Can you work these out from the model? Positions are in its coordinate system, mm. Coordinates: 2 decimals unless noted, no trailing zeros. Order: outer loops, then holes, each group sorted by start corner. A loop starts at its lowest first (then second) coordinate and runs counter-clockwise, first axis right, second up. Notation, with made-up numbers: M 29,-22.75 L 88,-22.75 A22 ccw 88,9.25 Z; hole C 66,60.5 d5. An arc over 180 degrees is marked long. Answer as CSV lines item,"result". Start each with the question number.
1. I need wall thicknesses on line 1 along Y through (x, z) = (-23, -36); line 2 along Z through (x, y) = (3.5, 2.15); line 3 along Z through (x, y) = (17, 0.6). Which ranges of each line are inside material? Lowest first, please. Write a range as from..to.
2. If we section it at A-A (x = -22): List the corners of the cut face in (y, z) for me, plus the area to 3 significant figures.
3. If we section it at B-B (y = 0.85): List the corners of the cut face in (x, z) for me.
```python
from build123d import *

# Parameters (mm, degrees)
SKETCH1_W               = 50
SKETCH1_H               = 80
BOSS_EXTRUDE1_DEPTH     = 5
CUT_EXTRUDE1_DEPTH      = 41
CUT_EXTRUDE1_DEPTH_BACK = 41
CUT_EXTRUDE2_DEPTH      = 26
CUT_EXTRUDE2_DEPTH_BACK = 26


with BuildPart() as part:
    # Sketch1 → Boss-Extrude1 (new body)
    with BuildSketch(Plane(origin=(0, 0, 0), x_dir=(1, 0, 0), z_dir=(0, 1, 0))):
        Rectangle(SKETCH1_W, SKETCH1_H)
    extrude(amount=BOSS_EXTRUDE1_DEPTH)

    # Sketch2 → Cut-Extrude1 (cut, two sides)
    with BuildSketch(Plane.XY) as cut_extrude1_sk:
        Polygon((-25, 0), (-20, 5), (-25, 5), align=None)
        Polygon((25, 0), (20, 5), (25, 5), align=None)
    extrude(amount=CUT_EXTRUDE1_DEPTH, mode=Mode.SUBTRACT)
    extrude(cut_extrude1_sk.sketch, amount=-CUT_EXTRUDE1_DEPTH_BACK, mode=Mode.SUBTRACT)

    # Sketch3 → Cut-Extrude2 (cut, two sides)
    with BuildSketch(Plane(origin=(0, 0, 0), x_dir=(0, 0, -1), z_dir=(1, 0, 0))) as cut_extrude2_sk:
        Polygon((-40, 0), (-35, 5), (-40, 5), align=None)
        Polygon((40, 0), (35, 5), (40, 5), align=None)
    extrude(amount=CUT_EXTRUDE2_DEPTH, mode=Mode.SUBTRACT)
    extrude(cut_extrude2_sk.sketch, amount=-CUT_EXTRUDE2_DEPTH_BACK, mode=Mode.SUBTRACT)


solid = part.part
```
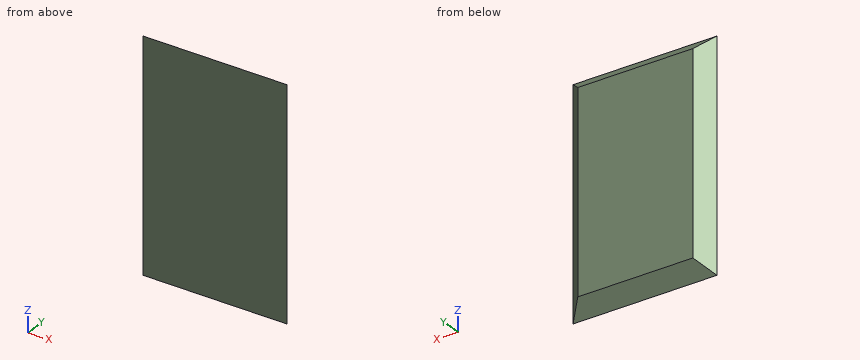
Solved:
1,line 1,"0..2"
1,line 2,"-37.85..37.85"
1,line 3,"-39.4..39.4"
2,outline,"M 0,-40 L 3,-37 L 3,37 L 0,40 Z"
2,area,"231 mm²"
3,outline,"M -24.15,-39.15 L 24.15,-39.15 L 24.15,39.15 L -24.15,39.15 Z"
